Check sheet for the modelled part. Datum: model origin and axes. Units: mm. A direction names the side the tool comes from. Round coordinates to 2 decimals unless told otherwise and drop trailing zeros. Write each loop counter-clockwise with the first axis right and the second up, starting at its lowest first coordinate (ties: lowest second). Pieces come first, ordered by that corner, then holes.
Item 1: Section check A-A, the plane z = 3.5. Record the cut outline in (x, y), plus the area to 3 significant figures.
Item 2: Section check D-D, the plane x = 0. Record the cut outline in (y, z).
Item 3: Material ranges on line 1 along X through (y, z) = (-1.75, 2.25); line 2 along Y through (x, z) = (0, 1); line 3 along Y through (x, z) = (0.25, 4.5), recorded low to high.
Item 4: Set-up check for faces 4 (the flat face through (6.133, -4, 2)), 5 (the flat face through (4, -4, 10.7)), 6 (the cylindrical face through (1.8, -5.4, 9.8)): record each of +Z, -Z, +X, -X, +Y, -Y from which the full face is reachable in a straight line by a thin tool's end or side.
Item 5: Section check B-B, the plane x = 3. Record the cut outline in (y, z), plus the area to 3 significant figures.
Item 6: Depth check by flat-ended pin: pin 1 (1 mm diameter, centred on x = -3.5, y = -7, fed in from +Z); pin 2 (1.5 mm diameter, centred on x = -5.5, y = -2.5, fed in from -Z). Enter the tip coordinate at first touch or a pass-through.
Item 7: Release check for a two-part mould opening along Y. For faces 1 (the cylindrical face through (-0.61, -2.45, 2.28)), 2 (the flat face through (0, -7.874, 4)), 3 (the flat face through (0, 0, 4)) record: pulls with the +Y half, pulls with the -Y half, needs draft (parallel to the pull), parting line crosses it, or undercut.
Item 8: Section check C-C, the plane y = -5. Record the cut outline in (x, z).
from build123d import *

# Parameters (mm, degrees)
F0_W     = 15.875
F0_H     = 9.525
F1_DEPTH = 7.874
F2_R     = 2.413
F3_DEPTH = 1.85
F4_W     = 12.827
F4_H     = 4.826
F4_R     = 1.524
F5_DEPTH = 6


with BuildPart() as f1:
    # F0 (on Front) → F1 (new body)
    with BuildSketch(Plane.XZ):
        with Locations((-0.280751, 4.087655)):
            Rectangle(F0_W, F0_H)
    extrude(amount=F1_DEPTH)

    # F2 (on face) → F3 (join)
    with BuildSketch(Plane.XY.offset(8.850155)):
        with Locations((-4.281251, -3.937)):
            Circle(F2_R)
        with Locations((3.719749, -3.937)):
            Circle(F2_R)
    extrude(amount=F3_DEPTH)

    # F4 (on face) → F5 (cut)
    with BuildSketch(Plane(origin=(0, 0, -0.674845), x_dir=(1, 0, 0), z_dir=(0, 0, -1))):
        with Locations((-0.280751, 3.937)):
            Rectangle(F4_W, F4_H)
        with Locations((-0.280751, 3.937)):
            Circle(F4_R, mode=Mode.SUBTRACT)
    extrude(amount=-F5_DEPTH, mode=Mode.SUBTRACT)


solid = f1.part
Values found:
1. outline: (-8.22, -7.87) - (7.66, -7.87) - (7.66, 0) - (-8.22, 0) - close; circle Ø3.05 at (-0.28, -3.94); hole (-6.69, -6.35) - (6.13, -6.35) - (6.13, -1.52) - (-6.69, -1.52) - close
1. area: 70.4 mm2
2. outline: (-7.87, -0.67) - (-6.35, -0.67) - (-6.35, 5.33) - (-5.43, 5.33) - (-5.43, -0.67) - (-2.44, -0.67) - (-2.44, 5.33) - (-1.52, 5.33) - (-1.52, -0.67) - (0, -0.67) - (0, 8.85) - (-7.87, 8.85) - close
3. line 1: x = -8.22 to -6.69, 6.13 to 7.66
3. line 2: y = -7.87 to -6.35, -5.43 to -2.44, -1.52 to 0
3. line 3: y = -7.87 to -6.35, -5.37 to -2.51, -1.52 to 0
4. face 4: -Z
4. face 5: +Z, +X, -X, +Y, -Y
4. face 6: +Z
5. outline: (-7.87, -0.67) - (-6.35, -0.67) - (-6.35, 5.33) - (-1.52, 5.33) - (-1.52, -0.67) - (0, -0.67) - (0, 8.85) - (-1.63, 8.85) - (-1.63, 10.7) - (-6.24, 10.7) - (-6.24, 8.85) - (-7.87, 8.85) - close
5. area: 54.6 mm2
6. pin 1: stops at z = 8.85
6. pin 2: stops at z = 5.33
7. face 1: undercut
7. face 2: pulls with the -Y half
7. face 3: pulls with the +Y half
8. outline: (-8.22, -0.67) - (-6.69, -0.67) - (-6.69, 5.33) - (-1.37, 5.33) - (-1.37, -0.67) - (0.81, -0.67) - (0.81, 5.33) - (6.13, 5.33) - (6.13, -0.67) - (7.66, -0.67) - (7.66, 8.85) - (5.89, 8.85) - (5.89, 10.7) - (1.55, 10.7) - (1.55, 8.85) - (-2.12, 8.85) - (-2.12, 10.7) - (-6.45, 10.7) - (-6.45, 8.85) - (-8.22, 8.85) - close
